Part model, mm, in its own coordinate system. Face numbers are marked on the shaded views. A direction names the side the tool comes from. Round coordinates to 2 decimals unless told otherwise and drop trailing zeros. Loops run counter-clockwise (first coordinate to the right, second up) from the corner with the lowest first, then second, coordinate; pieces in that order, holes last. Notation, with made-up numbers: (40, 5.5) - (46, 5.5) arc R32 cw to (46, 40.5) - close; hole circle Ø8 at (21, 47). An arc over 180 degrees is marked (long way). Put each result on its own line as item: value.
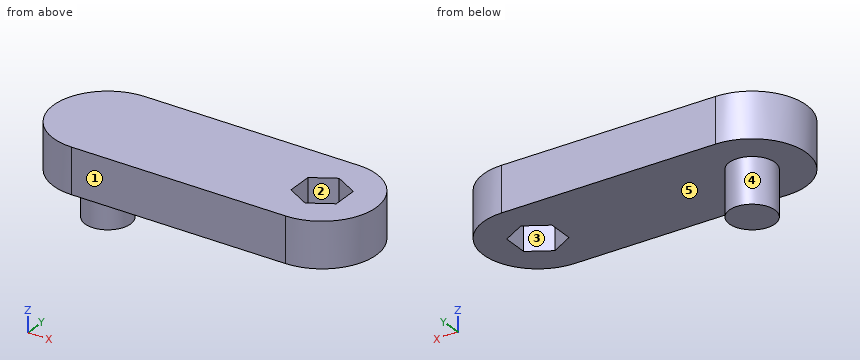
from build123d import *

# Parameters (mm, degrees)
EXTRUDE_1_DEPTH = 5
SKETCH_3_R      = 2.52
EXTRUDE_3_DEPTH = 5


with BuildPart() as part:
    # 草图1 → 凸台-拉伸1 (new body)
    with BuildSketch(Plane.XY):
        with BuildLine():
            Line((0, 6), (23.979571043, 6))
            ThreePointArc((23.979571043, 6), (29.979571043, 0), (23.979571043, -6))
            Line((23.979571043, -6), (0, -6))
            ThreePointArc((0, -6), (-6, 0), (0, 6))
        make_face()
        Polygon((26.50899235, -1.391172594), (26.449072504, 1.494956812), (23.919651197, 2.886129406), (21.450149737, 1.391172594), (21.510069583, -1.494956812), (24.039490889, -2.886129406), align=None, mode=Mode.SUBTRACT)
    extrude(amount=EXTRUDE_1_DEPTH)

    # 草图3 → 凸台-拉伸3 (add)
    with BuildSketch(Plane(origin=(0, 0, 0), x_dir=(-1, 0, 0), z_dir=(0, 0, -1))):
        with Locations(Location((0, 0, 0), (0, 0, 180))):
            Circle(SKETCH_3_R)
    extrude(amount=EXTRUDE_3_DEPTH)


solid = part.part
1. Pin check, flat tips, straight feed: P1, Ø1, axis at y = -0.5, z = 3.5, coming from the +X side; P2, Ø3, axis at x = 25.5, y = -4, coming from the -Z side; P3, Ø2, axis at y = 3.5, z = 2, coming from the -X side. Stop position of each tip, or through.
A:
P1: stops at x = 29.98
P2: stops at z = 0
P3: stops at x = -5.45
2. Band-saw the part on B-B (x = 17.5). List the corners of the cut face in (y, z).
A:
outline: (-6, 0) - (6, 0) - (6, 5) - (-6, 5) - close
3. Tool access for the marked faces 1 and 2: list every direction of +Z, -Z, +X, -X, +Y, -Y with a clear straight run to the whole face (end or side of a thin tool).
A:
face 1: +Z, -Z, +X, -X, -Y
face 2: +Z, -Z
4. Two-plate mould, pull along Y, no slides. Class the marked faces 3, 4 and 5: pulls with the +Y half, pulls with the -Y half, needs draft (parallel to the pull), parting line crosses it, or undercut.
A:
face 3: undercut
face 4: parting line crosses it
face 5: needs draft
5. Band-saw the part on D-D (y = -3.5). List the corners of the cut face in (x, z).
A:
outline: (-4.87, 0) - (28.85, 0) - (28.85, 5) - (-4.87, 5) - close
6. Band-saw the part on C-C (z = -4.5). List the corners of the cut face in (x, y).
A:
outline: circle Ø5.04 at (0, 0)
7. Band-saw the part on A-A (y = -1). List the corners of the cut face in (x, z), plus the area to 3 significant figures.
A:
outline: (-5.92, 0) - (-2.31, 0) - (-2.31, -5) - (2.31, -5) - (2.31, 0) - (21.5, 0) - (21.5, 5) - (-5.92, 5) - close; (26.5, 0) - (29.9, 0) - (29.9, 5) - (26.5, 5) - close
area: 177 mm²
8. Probe line 1 along Z through (x, y) = (27, -0.5); line 2 along X through (y, z) = (2.75, 3.25); line 3 along Y through (x, z) = (25, 1). List the from-to ranges inside material, lowest first. Write a range as [from, to].
A:
line 1: z = [0, 5]
line 2: x = [-5.33, 23.69], [24.17, 29.31]
line 3: y = [-5.91, -2.3], [2.29, 5.91]
